Source: CAD feature listing. Evaluate the final solid. Frame: model axes, mm. Face numbers are marked on the shaded views. A direction names the side the tool comes from. Round coordinates to 2 decimals unless told otherwise and drop trailing zeros. Write each loop counter-clockwise with the first axis right and the second up, starting at its lowest first coordinate (ties: lowest second). Pieces come first, ordered by that corner, then holes. Notation, with made-up numbers: M 34.5,73.25 L 58.5,73.25 A30 ccw 58.5,99.25 Z; hole C -28,10.25 d8. An arc over 180 degrees is marked long. Use a Markdown table: item, result.
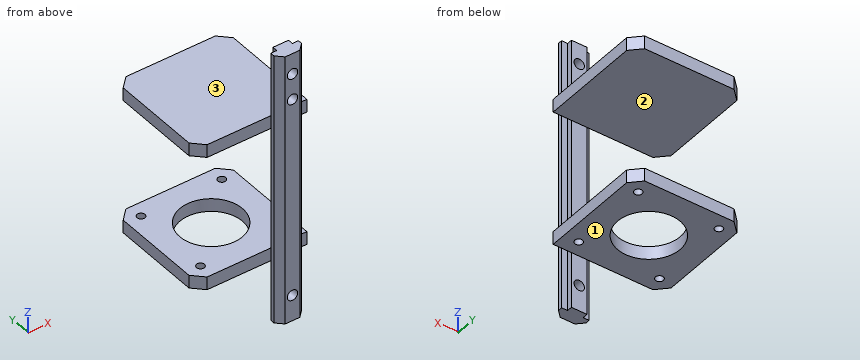
```python
from build123d import *

# Parameters (mm, degrees)
BOSS_EXTRUDE1_DEPTH        = 28.5
BOSS_EXTRUDE2_DEPTH        = 5
CHAMFER1_SIZE              = 4
LPATTERN1_COUNT            = 2
LPATTERN1_PITCH            = 52
CHAMFER1_OF_LPATTERN1_SIZE = 4
CUT_EXTRUDE1_REACH         = 79.984
SKETCH4_R                  = 12
SKETCH4_R_2                = 1.5
BOSS_EXTRUDE3_DEPTH        = 55
BOSS_EXTRUDE3_DEPTH_BACK   = 50
SKETCH6_R                  = 2
CUT_EXTRUDE2_DEPTH         = 77.534828673


with BuildPart() as part:
    # Sketch1 → Boss-Extrude1 (new, symmetric)
    with BuildSketch(Plane.XY):
        Polygon((-3, 0), (3, 0), (3, -2), (5.3, -2), (5.3, -3.62), (2.8, -6.1), (-2.8, -6.1), (-5.3, -3.62), (-5.3, -2), (-3, -2), align=None)
    extrude(amount=BOSS_EXTRUDE1_DEPTH, both=True)

    # Sketch2 → Boss-Extrude2 (add)
    with BuildSketch(Plane(origin=(0, 0, -28.5), x_dir=(-1, 0, 0), z_dir=(0, 0, -1))):
        Polygon((32.3, 0), (32.3, 42.3), (-10, 42.3), (-10, 0), (0, 0), align=None)
    boss_extrude2 = extrude(amount=-BOSS_EXTRUDE2_DEPTH)

    # Chamfer1
    chamfer1_edges = [part.edges().sort_by_distance(p)[0] for p in [
        (-32.3, 0, -26),
        (10, 42.3, -26),
        (-32.3, 42.3, -26),
    ]]
    chamfer(chamfer1_edges, length=CHAMFER1_SIZE)

    # LPattern1: Boss-Extrude2 ×2
    with Locations(*[(0, 0, i * LPATTERN1_PITCH) for i in range(1, LPATTERN1_COUNT)]):
        add(boss_extrude2)

    # Chamfer1 of LPattern1
    chamfer1_of_lpattern1_edges = [part.edges().sort_by_distance(p)[0] for p in [
        (-32.3, 0, 26),
        (10, 42.3, 26),
        (-32.3, 42.3, 26),
    ]]
    chamfer(chamfer1_of_lpattern1_edges, length=CHAMFER1_OF_LPATTERN1_SIZE)

    # Sketch4 → Cut-Extrude1 (cut, up to next)
    with BuildSketch(Plane(origin=(0, 0, -28.5), x_dir=(-1, 0, 0), z_dir=(0, 0, -1)), mode=Mode.PRIVATE) as cut_extrude1_sk1:
        with Locations((11.15, 21.15)):
            Circle(SKETCH4_R)
    cut_extrude1_tool1 = extrude(cut_extrude1_sk1.sketch, amount=-CUT_EXTRUDE1_REACH, mode=Mode.PRIVATE) & part.part
    # Sketch4 → Cut-Extrude1 (cut, up to next)
    with BuildSketch(Plane(origin=(0, 0, -28.5), x_dir=(-1, 0, 0), z_dir=(0, 0, -1)), mode=Mode.PRIVATE) as cut_extrude1_sk2:
        with Locations((26.65, 36.65)):
            Circle(SKETCH4_R_2)
    cut_extrude1_tool2 = extrude(cut_extrude1_sk2.sketch, amount=-CUT_EXTRUDE1_REACH, mode=Mode.PRIVATE) & part.part
    # Sketch4 → Cut-Extrude1 (cut, up to next)
    with BuildSketch(Plane(origin=(0, 0, -28.5), x_dir=(-1, 0, 0), z_dir=(0, 0, -1)), mode=Mode.PRIVATE) as cut_extrude1_sk3:
        with Locations((-4.35, 36.65)):
            Circle(SKETCH4_R_2)
    cut_extrude1_tool3 = extrude(cut_extrude1_sk3.sketch, amount=-CUT_EXTRUDE1_REACH, mode=Mode.PRIVATE) & part.part
    # Sketch4 → Cut-Extrude1 (cut, up to next)
    with BuildSketch(Plane(origin=(0, 0, -28.5), x_dir=(-1, 0, 0), z_dir=(0, 0, -1)), mode=Mode.PRIVATE) as cut_extrude1_sk4:
        with Locations((-4.35, 5.65)):
            Circle(SKETCH4_R_2)
    cut_extrude1_tool4 = extrude(cut_extrude1_sk4.sketch, amount=-CUT_EXTRUDE1_REACH, mode=Mode.PRIVATE) & part.part
    # Sketch4 → Cut-Extrude1 (cut, up to next)
    with BuildSketch(Plane(origin=(0, 0, -28.5), x_dir=(-1, 0, 0), z_dir=(0, 0, -1)), mode=Mode.PRIVATE) as cut_extrude1_sk5:
        with Locations((26.65, 5.65)):
            Circle(SKETCH4_R_2)
    cut_extrude1_tool5 = extrude(cut_extrude1_sk5.sketch, amount=-CUT_EXTRUDE1_REACH, mode=Mode.PRIVATE) & part.part
    add(cut_extrude1_tool1.solids().sort_by_distance((-11.15, 21.15, -28.5))[0], mode=Mode.SUBTRACT)
    add(cut_extrude1_tool2.solids().sort_by_distance((-26.65, 36.65, -28.5))[0], mode=Mode.SUBTRACT)
    add(cut_extrude1_tool3.solids().sort_by_distance((4.35, 36.65, -28.5))[0], mode=Mode.SUBTRACT)
    add(cut_extrude1_tool4.solids().sort_by_distance((4.35, 5.65, -28.5))[0], mode=Mode.SUBTRACT)
    add(cut_extrude1_tool5.solids().sort_by_distance((-26.65, 5.65, -28.5))[0], mode=Mode.SUBTRACT)

    # Sketch5 → Boss-Extrude3 (add, two sides: drawn at the far end of the back side and taken through both)
    with BuildSketch(Plane.XY.offset(-BOSS_EXTRUDE3_DEPTH_BACK)):
        Polygon((-3, -2), (-5.3, -2), (-5.3, -3.62), (-2.8, -6.1), (2.8, -6.1), (5.3, -3.62), (5.3, -2), (3, -2), (3, 0), (-3, 0), align=None)
    extrude(amount=BOSS_EXTRUDE3_DEPTH + BOSS_EXTRUDE3_DEPTH_BACK)

    # Sketch6 → Cut-Extrude2 (cut, through all)
    with BuildSketch(Plane(origin=(0, 0, 0), x_dir=(1, 0, 0), z_dir=(0, 1, 0))):
        with Locations(Location((0, 40, 0), (0, 0, 270))):
            Circle(SKETCH6_R)
        with Locations(Location((0, -37, 0), (0, 0, 270))):
            Circle(SKETCH6_R)
        with Locations(Location((0, -47, 0), (0, 0, 270))):
            Circle(SKETCH6_R)
    extrude(amount=-CUT_EXTRUDE2_DEPTH, mode=Mode.SUBTRACT)


solid = part.part
```
Q1. Section D-D on x = -11.15. Return loops of the section in (y, z).
Results are:
| item | result |
|---|---|
| outline | M 0,-28.5 L 9.15,-28.5 L 9.15,-23.5 L 0,-23.5 Z; M 0,23.5 L 42.3,23.5 L 42.3,28.5 L 0,28.5 Z; M 33.15,-28.5 L 42.3,-28.5 L 42.3,-23.5 L 33.15,-23.5 Z |
Q2. Line query: L1, parallel to X at y = -2.25, z = 47; L2, parallel to X at y = -1, z = 47; L3, parallel to Z at x = 2, y = 15. Output: solid intervals per line, ascending.
Results are:
| item | result |
|---|---|
| L1 | -5.3 to -2, 2 to 5.3 |
| L2 | -3 to -2, 2 to 3 |
| L3 | -28.5 to -23.5, 23.5 to 28.5 |
Q3. Section B-B on z = 37. Return loops of the section in (x, y), plus the area to 3 significant figures.
Results are:
| item | result |
|---|---|
| outline | M -5.3,-3.62 L -2.8,-6.1 L -2,-6.1 L -2,0 L -3,0 L -3,-2 L -5.3,-2 Z; M 2,-6.1 L 2.8,-6.1 L 5.3,-3.62 L 5.3,-2 L 3,-2 L 3,0 L 2,0 Z |
| area | 24.9 mm^2 |
Q4. Reachability of the marked faces 1, 2 and 3 from +Z, -Z, +X, -X, +Y, -Y: full face, straight path, thin tool, end or side. Return the list, or none.
Results are:
| item | result |
|---|---|
| face 1 | -Z, +X, -X, +Y |
| face 2 | +X, -X, +Y |
| face 3 | +Z, +X, -X, +Y |
Q5. Section A-A on x = 7.5. Return loops of the section in (y, z).
Results are:
| item | result |
|---|---|
| outline | M 0,-28.5 L 40.8,-28.5 L 40.8,-23.5 L 0,-23.5 Z; M 0,23.5 L 40.8,23.5 L 40.8,28.5 L 0,28.5 Z |
Q6. First-contact query: pin 1 Ø2.5 at (x, z) = (-11, -25) entering from -Y; pin 2 Ø1 at (y, z) = (-1, 20) entering from -X; pin 3 Ø0.5 at (y, z) = (-2.5, -17) entering from +X; pin 4 Ø1 at (y, z) = (1, 34) entering from -X. Flat tips, straight axial feed; report the tip coordinate or a pass-through.
Results are:
| item | result |
|---|---|
| pin 1 | y = 0 |
| pin 2 | x = -3 |
| pin 3 | x = 5.3 |
| pin 4 | through |
Q7. Section C-C on y = 18.5. Return loops of the section in (x, z).
Results are:
| item | result |
|---|---|
| outline | M -32.3,-28.5 L -22.85,-28.5 L -22.85,-23.5 L -32.3,-23.5 Z; M -32.3,23.5 L 10,23.5 L 10,28.5 L -32.3,28.5 Z; M 0.55,-28.5 L 10,-28.5 L 10,-23.5 L 0.55,-23.5 Z |
